```python
from build123d import *

# Parameters (mm, degrees)
F0_W     = 3.175
F0_H     = 152.4
F1_DEPTH = 114.3
F2_W     = 127
F2_H     = 98.425
F3_DEPTH = 25.4
F4_W     = 119.929246
F4_H     = 3.175
F5_DEPTH = 12.7
F7_DEPTH = 25.4
F9_DEPTH = 25.4


with BuildPart() as f1:
    # F0 (on Top) → F1 (new body)
    with BuildSketch(Plane.XY):
        Rectangle(F0_W, F0_H)
    extrude(amount=F1_DEPTH)

    # F2 (on face) → F3 (cut)
    with BuildSketch(Plane.YZ.offset(1.5875)):
        with Locations((0, 57.15)):
            Rectangle(F2_W, F2_H)
    extrude(amount=-F3_DEPTH, mode=Mode.SUBTRACT)

    # F4 (on face) → F5 (join)
    with BuildSketch(Plane.YZ.offset(1.5875)):
        with Locations((2.900731, 112.7125)):
            Rectangle(F4_W, F4_H)
    extrude(amount=F5_DEPTH)

    # F6 (on face) → F7 (cut)
    with BuildSketch(Plane.XY.offset(114.3)):
        Polygon((14.2875, 62.865354), (1.5875, 62.865354), (14.2875, 59.108607), align=None)
        Polygon((14.2875, -43.201216), (1.5875, -57.063892), (14.2875, -57.063892), align=None)
    extrude(amount=-F7_DEPTH, mode=Mode.SUBTRACT)

    # F8 (on face) → F9 (cut)
    with BuildSketch(Plane.XY.offset(114.3)):
        with BuildLine():
            ThreePointArc((11.1125, 48.286981), (10.182564, 50.532045), (7.9375, 51.461981))
            Line((7.9375, 51.461981), (7.9375, 45.111981))
            ThreePointArc((7.9375, 45.111981), (10.182564, 46.041917), (11.1125, 48.286981))
        make_face()
        with BuildLine():
            ThreePointArc((11.1125, -37.432554), (10.182564, -35.18749), (7.9375, -34.257554))
            Line((7.9375, -34.257554), (7.9375, -40.607554))
            ThreePointArc((7.9375, -40.607554), (10.182564, -39.677618), (11.1125, -37.432554))
        make_face()
        with BuildLine():
            Line((7.9375, -40.607554), (7.9375, -34.257554))
            ThreePointArc((7.9375, -34.257554), (4.7625, -37.432554), (7.9375, -40.607554))
        make_face()
        with BuildLine():
            ThreePointArc((11.1125, 5.427213), (10.182564, 7.672277), (7.9375, 8.602213))
            Line((7.9375, 8.602213), (7.9375, 2.252213))
            ThreePointArc((7.9375, 2.252213), (10.182564, 3.182149), (11.1125, 5.427213))
        make_face()
        with BuildLine():
            Line((7.9375, 2.252213), (7.9375, 8.602213))
            ThreePointArc((7.9375, 8.602213), (4.7625, 5.427213), (7.9375, 2.252213))
        make_face()
        with BuildLine():
            Line((7.9375, 45.111981), (7.9375, 51.461981))
            ThreePointArc((7.9375, 51.461981), (4.7625, 48.286981), (7.9375, 45.111981))
        make_face()
    extrude(amount=-F9_DEPTH, mode=Mode.SUBTRACT)


solid = f1.part
```
Geometry check sheet. Reference: the model listing, model coordinates, mm. A direction names the side the tool comes from. Coordinates: 2 decimals unless noted, no trailing zeros. Order: outer loops, then holes, each group sorted by start corner. A loop starts at its lowest first (then second) coordinate and runs counter-clockwise, first axis right, second up.
Item 1: Section check B-B (z = 69.5). Enter the section's corners in (x, y).
Item 2: Section check C-C (x = 0). Enter the section's corners in (y, z), plus the area to 3 significant figures.
Item 3: Mould release check, pull along Y, two halves, no side actions. Record for faces 4 (the flat face through (0, 1, 0)), 5 (the flat face through (8.026, -50.036, 112.735)), 6 (the flat face through (0, -1, 106.362)), 7 (the flat face through (0, -63.5, 56)): released by +Y, released by -Y, zero draft, split by the parting line, or undercut.
Item 4: Tool access check on faces 1 (the flat face through (-1.588, -1, 6)), 2 (the flat face through (0, 63.5, 56)), 3 (the flat face through (8, 2, 111.125)). Record the directions out of +Z, -Z, +X, -X, +Y, -Y that give a thin tool (end or side, any length) a straight path to the whole face; none if there is none.
Item 5: Scan lines: line 1 along Y through (x, z) = (1.25, 11.5); line 2 along Z through (x, y) = (1.5, -60.5); line 3 along Z through (x, y) = (10.75, 7.5) (3 decimals). Record each from-to range of solid material in increasing order.
Item 6: Depth check by flat-ended pin: pin 1 (3 mm diameter, centred on x = 5, z = 72, fed in from -Y); pin 2 (4 mm diameter, centred on x = 9.5, y = -3.5, fed in from -Z) (3 decimals). Enter the tip coordinate at first touch or a pass-through.
Item 7: Section check D-D (y = -46). Enter the section's corners in (x, z) (1 decimal).
Item 8: Section check A-A (y = -25.5). Enter the section's corners in (x, z) (1 decimal).
Check sheet entries:
1. outline: (-1.59, -76.2) - (1.59, -76.2) - (1.59, -63.5) - (-1.59, -63.5) - close; (-1.59, 63.5) - (1.59, 63.5) - (1.59, 76.2) - (-1.59, 76.2) - close
2. outline: (-76.2, 0) - (76.2, 0) - (76.2, 114.3) - (-76.2, 114.3) - close; hole (-63.5, 7.94) - (63.5, 7.94) - (63.5, 106.36) - (-63.5, 106.36) - close
2. area: 4,920 mm2
3. face 4: zero draft
3. face 5: released by -Y
3. face 6: undercut
3. face 7: undercut
4. face 1: +Z, -Z, -X, +Y, -Y
4. face 2: +X, -X
4. face 3: -Z, +X, +Y, -Y
5. line 1: y = -76.2 to -63.5, 63.5 to 76.2
5. line 2: z = 0 to 7.94, 106.36 to 114.3
5. line 3: z = 111.125 to 114.3
6. pin 1: passes through
6. pin 2: stops at z = 111.125
7. outline: (-1.6, 0) - (1.6, 0) - (1.6, 7.9) - (-1.6, 7.9) - close; (-1.6, 106.4) - (1.6, 106.4) - (1.6, 111.1) - (11.7, 111.1) - (11.7, 114.3) - (-1.6, 114.3) - close
8. outline: (-1.6, 0) - (1.6, 0) - (1.6, 7.9) - (-1.6, 7.9) - close; (-1.6, 106.4) - (1.6, 106.4) - (1.6, 111.1) - (14.3, 111.1) - (14.3, 114.3) - (-1.6, 114.3) - close
